Answer from the drawing. Dimensions are ordinates in mm from the lowest x, y and z of the part. A direction names the side the tool comes from. Coordinates: 2 decimals unless noted, no trailing zeros. Loops run counter-clockwise (first coordinate to the right, second up) from the corner with the lowest first, then second, coordinate; pieces in that order, holes last. Notation, with made-up numbers: (83, -17) - (119, -17) arc R22 cw to (119, 9) - close; hole circle Ø11 at (-25, 80). An arc over 180 degrees is marked (long way). Use one line per item in the form item = value. Start each with the question number.
1) A cutting plane is placed at A-A (z = 8.75). Give the vertices of the cut face in (x, y) (1 decimal).
2) The mould has two halves that part along X. Classify the marked faces 1, 2 and 3: released by +X, released by -X, zero draft, split by the parting line, or undercut.
3) Each of these flat-tipped pins is pushed along its axis until it touches: P1, Ø1.5, axis at x = 8, y = 2, coming from the -Z side; P2, Ø1.6, axis at x = 4.5, y = 4.5, coming from the +Z side. Where does it stop, or does it pass through?
4) A cutting plane is placed at B-B (x = 7). Give the vertices of the cut face in (y, z) (1 decimal).
5) Consider line 1 (X direction, y = 6.5, z = 7) (1 decimal); line 2 (Y direction, x = 2.5, z = 8) (1 decimal); line 3 (Z direction, x = 8, y = 2). Determine where each line is inside the solid, lowest interval first.
6) Which of the six approach directions +Z, -Z, +X, -X, +Y, -Y give full straight-line access (tool end or side, diameter ignored) to the marked faces 4, 5 and 6?
7) A cutting plane is placed at C-C (y = 3). Give the vertices of the cut face in (x, z) (1 decimal).
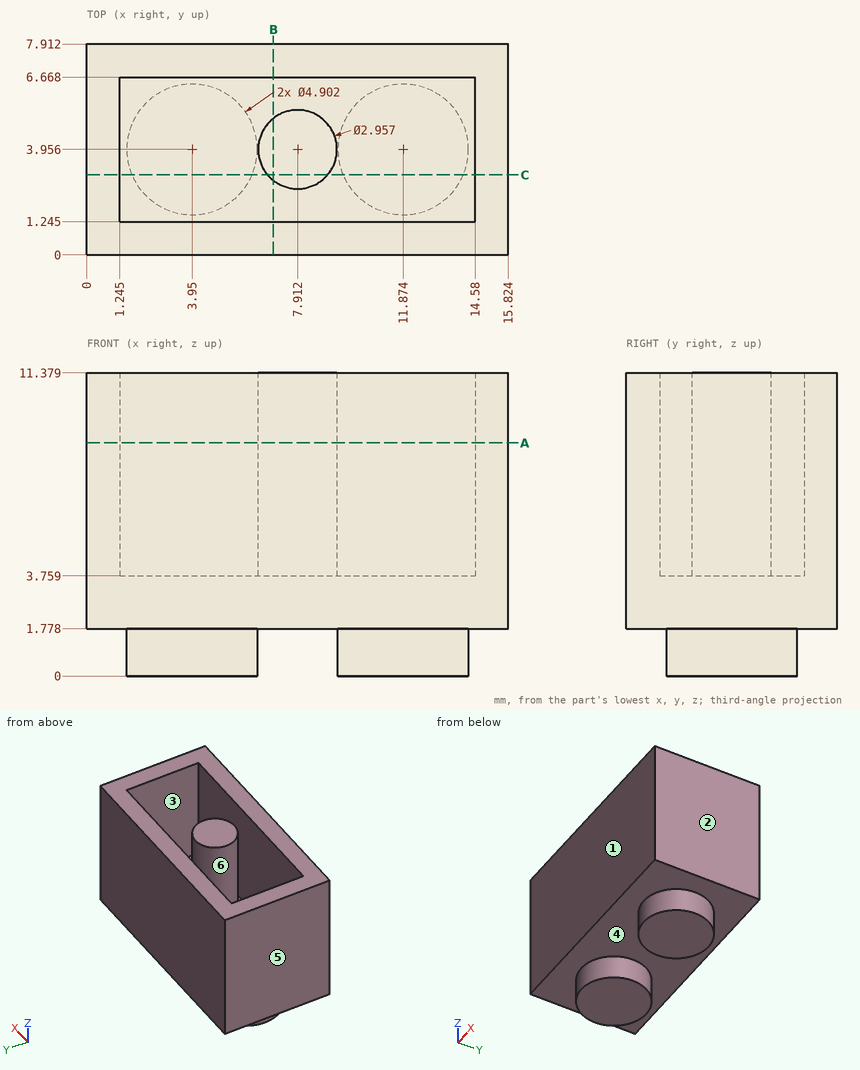
Found:
q1.outline = (0, 0) - (15.8, 0) - (15.8, 7.9) - (0, 7.9) - close; circle Ø3 at (7.9, 4); hole (1.2, 1.2) - (14.6, 1.2) - (14.6, 6.7) - (1.2, 6.7) - close
q2.face_1 = zero draft
q2.face_2 = released by +X
q2.face_3 = undercut
q3.P1 = 1.78
q3.P2 = 3.76
q4.outline = (0, 1.8) - (7.9, 1.8) - (7.9, 11.4) - (6.7, 11.4) - (6.7, 3.8) - (5.1, 3.8) - (5.1, 11.4) - (2.8, 11.4) - (2.8, 3.8) - (1.2, 3.8) - (1.2, 11.4) - (0, 11.4) - close
q5.line_1 = 0 to 1.2, 14.6 to 15.8
q5.line_2 = 0 to 1.2, 6.7 to 7.9
q5.line_3 = 1.78 to 3.76
q6.face_4 = -Z
q6.face_5 = +Z, -Z, -X, +Y, -Y
q6.face_6 = +Z
q7.outline = (0, 1.8) - (1.7, 1.8) - (1.7, 0) - (6.2, 0) - (6.2, 1.8) - (9.6, 1.8) - (9.6, 0) - (14.1, 0) - (14.1, 1.8) - (15.8, 1.8) - (15.8, 11.4) - (14.6, 11.4) - (14.6, 3.8) - (9, 3.8) - (9, 11.4) - (6.8, 11.4) - (6.8, 3.8) - (1.2, 3.8) - (1.2, 11.4) - (0, 11.4) - close
